```python
from build123d import *

# Parameters (mm, degrees)
BOSS_EXTRUDE1_DEPTH = 21
CUT_EXTRUDE1_DEPTH  = 60
CUT_EXTRUDE1_DRAFT  = -1
CUT_EXTRUDE2_REACH  = 112.553
BOSS_EXTRUDE2_START = 4
BOSS_EXTRUDE2_DEPTH = 4


with BuildPart() as part:
    # Sketch1 → Boss-Extrude1 (new, symmetric)
    with BuildSketch(Plane(origin=(0, 0, 0), x_dir=(0, 0, -1), z_dir=(1, 0, 0))):
        Polygon((0, 0), (-100, 0), (-100, 10), (-60, 10), (-60, 31), (-46.752018394, 52.201202404), (0, 22.987298969), align=None)
    extrude(amount=BOSS_EXTRUDE1_DEPTH, both=True)


with BuildPart() as cut_extrude1_tool:
    # Sketch2 → Cut-Extrude1 (with draft: the straight prism first)
    with BuildSketch(Plane(origin=(0, 35.669068614, 57.082442121), x_dir=(1, 0, 0), z_dir=(0, 0.5299192642331993, 0.8480480961564296))):
        Polygon((-5.821903288, 20.603497628), (-11.5, 12.494335127), (11.5, 12.494335127), (5.821903288, 20.603497628), align=None)
    extrude(amount=-CUT_EXTRUDE1_DEPTH)
    # Cut-Extrude1: the draft: its side faces are tilted about the plane it starts from
    cut_extrude1_sides = [cut_extrude1_tool.faces().sort_by_distance(p)[0] for p in [
        (-8.660951644, 33.805767714, 22.871409646),
        (0, 30.367287804, 25.020010359),
        (8.660951644, 33.805767714, 22.871409646),
        (0, 37.244247624, 20.722808933),
    ]]
    draft(cut_extrude1_sides, Plane(origin=(0, 35.669068614, 57.082442121), x_dir=(1, 0, 0), z_dir=(0, 0.5299192642331993, 0.8480480961564296)), CUT_EXTRUDE1_DRAFT)


with BuildPart() as part_1:
    add(part.part)

    # Cut-Extrude1: cut by cut_extrude1_tool
    add(cut_extrude1_tool.part, mode=Mode.SUBTRACT)

    # Sketch3 → Cut-Extrude2 (cut, up to next)
    with BuildSketch(Plane(origin=(0, 10, 0), x_dir=(1, 0, 0), z_dir=(0, 1, 0)), mode=Mode.PRIVATE) as cut_extrude2_sk1:
        with BuildLine():
            Line((9.5, -78), (-9.5, -78))
            ThreePointArc((-9.5, -78), (-14.5, -83), (-9.5, -88))
            Line((-9.5, -88), (9.5, -88))
            ThreePointArc((9.5, -88), (14.5, -83), (9.5, -78))
        make_face()
    cut_extrude2_tool1 = extrude(cut_extrude2_sk1.sketch, amount=-CUT_EXTRUDE2_REACH, mode=Mode.PRIVATE) & part_1.part
    # Sketch3 → Cut-Extrude2 (cut, up to next)
    with BuildSketch(Plane(origin=(0, 10, 0), x_dir=(1, 0, 0), z_dir=(0, 1, 0)), mode=Mode.PRIVATE) as cut_extrude2_sk2:
        with BuildLine():
            ThreePointArc((-18, -100), (-20.121320344, -99.121320344), (-21, -97))
            Line((-21, -97), (-21, -100))
            Line((-21, -100), (-18, -100))
        make_face()
    cut_extrude2_tool2 = extrude(cut_extrude2_sk2.sketch, amount=-CUT_EXTRUDE2_REACH, mode=Mode.PRIVATE) & part_1.part
    # Sketch3 → Cut-Extrude2 (cut, up to next)
    with BuildSketch(Plane(origin=(0, 10, 0), x_dir=(1, 0, 0), z_dir=(0, 1, 0)), mode=Mode.PRIVATE) as cut_extrude2_sk3:
        with BuildLine():
            ThreePointArc((21, -97), (20.121320344, -99.121320344), (18, -100))
            Line((18, -100), (21, -100))
            Line((21, -100), (21, -97))
        make_face()
    cut_extrude2_tool3 = extrude(cut_extrude2_sk3.sketch, amount=-CUT_EXTRUDE2_REACH, mode=Mode.PRIVATE) & part_1.part
    add(cut_extrude2_tool1.solids().sort_by_distance((0, 10, 83))[0], mode=Mode.SUBTRACT)
    add(cut_extrude2_tool2.solids().sort_by_distance((-20.329896, 10, 99.329896))[0], mode=Mode.SUBTRACT)
    add(cut_extrude2_tool3.solids().sort_by_distance((20.329896, 10, 99.329896))[0], mode=Mode.SUBTRACT)

    # Sketch3_3 → Boss-Extrude2 (add)
    with BuildSketch(Plane(origin=(0, 10, 0), x_dir=(1, 0, 0), z_dir=(0, 1, 0)).offset(BOSS_EXTRUDE2_START)):
        with BuildLine():
            Line((-9.5, -76), (9.5, -76))
            ThreePointArc((9.5, -76), (16.5, -83), (9.5, -90))
            Line((9.5, -90), (-9.5, -90))
            ThreePointArc((-9.5, -90), (-16.5, -83), (-9.5, -76))
        make_face()
        with BuildLine():
            ThreePointArc((9.5, -88), (14.5, -83), (9.5, -78))
            Line((9.5, -78), (-9.5, -78))
            ThreePointArc((-9.5, -78), (-14.5, -83), (-9.5, -88))
            Line((-9.5, -88), (9.5, -88))
        make_face(mode=Mode.SUBTRACT)
    extrude(amount=-BOSS_EXTRUDE2_DEPTH)


solid = part_1.part
```
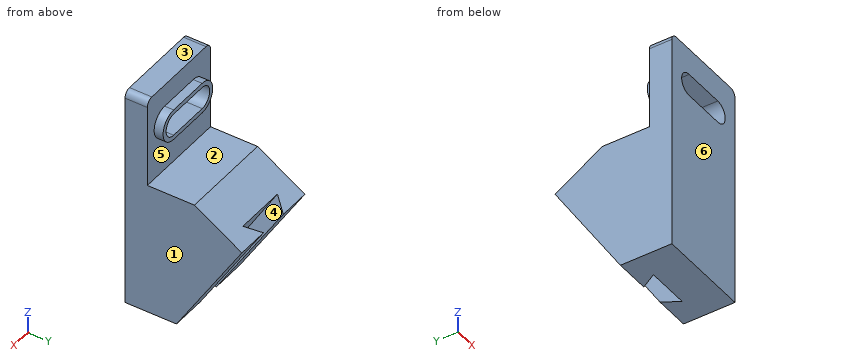
Could you check a few things on this model? Use its own coordinates, in mm. Face numbers are marked on the shaded views. A direction names the side the tool comes from. Give positions to 0.01 mm unless a question says otherwise; leave off trailing zeros. Write each loop counter-clockwise with the first axis right and the second up, starting at its lowest first coordinate (ties: lowest second). Pieces come first, ordered by that corner, then holes. Notation, with made-up numbers: (-12, -5) -> (38, -5) arc R19 ccw to (38, 2) -> close; hole circle Ø7 at (31, 0). An arc over 180 degrees is marked (long way). Write each question's results on one line, items separated by ' | '.
1. On a 3-axis mill with a long thin cutter (end or side, diameter ignored), from which of +Z, -Z, +X, -X, +Y, -Y can I reach the whole of each face in a straight line? I mean the marked faces 1 and 2. Say none if no direction works.
Check sheet entries:
face 1: +Z, -Z, +X, +Y, -Y | face 2: +X, -X, +Y
2. I want a section at A-A, the plane z = 83. Write out the boundary of the cut face in (x, y), then the cut area to 3 significant figures.
Check sheet entries:
outline: (-21, 0) -> (-14.5, 0) -> (-14.5, 14) -> (-16.5, 14) -> (-16.5, 10) -> (-21, 10) -> close; (14.5, 0) -> (21, 0) -> (21, 10) -> (16.5, 10) -> (16.5, 14) -> (14.5, 14) -> close | area: 146 mm²
3. I need wall thicknesses on L1, parallel to Z at x = 7, y = 4.5; L2, parallel to Y at x = -7.5, z = 65.5; L3, parallel to Z at x = 13, y = 16.5. Which ranges of each line are inside material? Lowest first, please.
Check sheet entries:
L1: z = 0 to 78, 88 to 100 | L2: y = 0 to 10 | L3: z = 0 to 60
4. If we mould it in two halves opening along Z, with no side actions, what happens to the marked faces 3, 4, 5 and 6? For each: released by +Z, released by -Z, zero draft, split by the parting line, or undercut.
Check sheet entries:
face 3: released by +Z | face 4: undercut | face 5: undercut | face 6: zero draft
5. I want a section at B-B, the plane y = 9. Write out the boundary of the cut face in (x, z), then the cut area to 3 significant figures.
Check sheet entries:
outline: (-21, 0) -> (21, 0) -> (21, 97) arc R3 ccw to (18, 100) -> (-18, 100) arc R3 ccw to (-21, 97) -> close; hole (-9.5, 78) -> (9.5, 78) arc R5 ccw to (9.5, 88) -> (-9.5, 88) arc R5 ccw to start | area: 3,930 mm²
6. I want a section at D-D, the plane x = 8. Write out the boundary of the cut face in (y, z), then the cut area to 3 significant figures.
Check sheet entries:
outline: (0, 0) -> (15.94, 0) -> (46.26, 50.46) -> (31, 60) -> (10, 60) -> (10, 76) -> (14, 76) -> (14, 78) -> (0, 78) -> close; (0, 88) -> (14, 88) -> (14, 90) -> (10, 90) -> (10, 100) -> (0, 100) -> close; (18.56, 0) -> (22.99, 0) -> (52.2, 46.75) -> (50.5, 47.81) -> close | area: 2,410 mm²
7. I want a section at C-C, the plane x = 12.5. Write out the boundary of the cut face in (y, z), then the cut area to 3 significant figures.
Check sheet entries:
outline: (0, 0) -> (22.99, 0) -> (52.2, 46.75) -> (31, 60) -> (10, 60) -> (10, 76.68) -> (14, 76.68) -> (14, 79) -> (0, 79) -> close; (0, 87) -> (14, 87) -> (14, 89.32) -> (10, 89.32) -> (10, 100) -> (0, 100) -> close | area: 2,650 mm²
8. Will these pins go through, and if not, where does the flat tip stop? pin 1 Ø3 at (x, y) = (0.5, 12) entering from +Z; pin 2 Ø11 at (x, z) = (-1.5, 83) entering from +Y; pin 3 Ø6 at (x, y) = (-5, 27) entering from -Z.
Check sheet entries:
pin 1: stops at z = 90 | pin 2: stops at y = 14 | pin 3: stops at z = 1.68
